Geometry check sheet. Reference: the model listing, model coordinates, mm. A direction names the side the tool comes from. Give positions to 0.01 mm unless a question says otherwise; leave off trailing zeros. Order: outer loops, then holes, each group sorted by start corner. A loop starts at its lowest first (then second) coordinate and runs counter-clockwise, first axis right, second up. Notation, with made-up numbers: (85, 47) - (124, 47) arc R36 ccw to (124, 85) - close; hole circle Ø6 at (31.25, -20.5). An arc over 180 degrees is marked (long way). Put each result on its own line as item: value. Start each with the question number.
Autodesk Inventor part; units mm, degrees
ref_plane "YZ Plane" through (0, 0, 0) normal (1, 0, 0) x (0, 1, 0)
ref_plane "XZ Plane" through (0, 0, 0) normal (0, 1, 0) x (-1, 0, 0)
ref_plane "XY Plane" through (0, 0, 0) normal (0, 0, 1) x (1, 0, 0)
sketch "Sketch1" plane through (0, 0, 0) normal (0, 0, 1) x (1, 0, 0)
  circle A0 centre (0, 0) radius 4
  circle A1 centre (0, 0) radius 50
  circle A2 centre (0, 0) radius 38
  dimension "d0" = 8
  dimension "d1" = 100
  dimension "d2" = 12
extrude "Extrusion1" add sketch "Sketch1" along normal blind 10 contours A1
sketch "Sketch2" plane through (0, 0, 10) normal (0, 0, 1) x (1, 0, 0)
  circle A0 centre (0, 0) radius 50
  circle A1 centre (0, 0) radius 4
  dimension "d5" = 8
  dimension "d6" = 100
sketch "Sketch3" plane through (0, 0, 10) normal (0, 0, 1) x (1, 0, 0)
  point P0 (0, 0)
extrude "Extrusion2" add sketch "Sketch2" along normal blind 6
sketch "Sketch4" plane through (0, 0, 16) normal (0, 0, 1) x (1, 0, 0)
  circle A0 centre (0, 0) radius 38
  circle A1 centre (0, 0) radius 50
  dimension "d9" = 76
  dimension "d10" = 100
extrude "Extrusion3" add sketch "Sketch4" along normal blind 10
sketch "Sketch5" plane through (0, 0, 16) normal (0, 0, 1) x (1, 0, 0)
  circle A0 centre (0, 0) radius 4
  circle A1 centre (0, 0) radius 6
  dimension "d13" = 8
  dimension "d14" = 12
extrude "Extrusion4" add sketch "Sketch5" along normal blind 20
properties part number "100mm wheel"
Item 1: Set-up check for faces 5 (the face through (-6, 0, 26)), 6 (the face through (17.535, 33.713, 4.93)), 7 (the face through (11, 37, 0)): record each of +Z, -Z, +X, -X, +Y, -Y from which the full face is reachable in a straight line by a thin tool's end or side.
Item 2: Cross-section at B-B (z = 22.5). Enter the section's corners in (x, y), and give its area (3 significant figures).
Item 3: Thickness scan on line 1 along Y through (x, z) = (0, 19.75); line 2 along Y through (x, z) = (0, 7.5); line 3 along Y through (x, z) = (0, 28). Record the ranges inside material, lowest first.
Item 4: Cross-section at D-D (y = 26.5). Enter the section's corners in (x, z), and give its area (3 significant figures).
Item 5: Release check for a two-part mould opening along Y. For faces 1 (the face through (17.535, 33.713, 20.93)), 2 (the face through (11, 37, 26)), 3 (the face through (47.69, -15.02, 12.82)), 4 (the face through (-1, -8, 10)) record: +Y half, -Y half, draft (parallel to the pull), parting line (faces both ways), or undercut.
Item 6: Cross-section at C-C (z = 7.5). Enter the section's corners in (x, y), and give its area (3 significant figures).
Item 7: Cross-section at A-A (x = 0). Enter the section's corners in (y, z), and give its area (3 significant figures).
Item 8: Gauge pin test, flat ends, axial feed: pin 1 Ø2 at (y, z) = (-23, 14) entering from +X; pin 2 Ø10 at (x, y) = (-27, -2.5) entering from -Z; pin 3 Ø6 at (x, z) = (6.5, 7.5) entering from +Y; pin 4 Ø7 at (x, y) = (0, 0) entering from +Z. Record the tip position at first contact, or that the pin passes through.
Recorded:
1. face 5: +Z
1. face 6: -Z
1. face 7: -Z, +X, -X, +Y, -Y
2. outline: circle Ø100 at (0, 0); circle Ø12 at (0, 0); hole circle Ø76 at (0, 0); hole circle Ø8 at (0, 0)
2. area: 3,380 mm^2
3. line 1: y = -50 to -38, -6 to -4, 4 to 6, 38 to 50
3. line 2: y = -50 to -38, 38 to 50
3. line 3: y = -6 to -4, 4 to 6
4. outline: (-42.4, 0) - (-27.24, 0) - (-27.24, 10) - (27.24, 10) - (27.24, 0) - (42.4, 0) - (42.4, 26) - (27.24, 26) - (27.24, 16) - (-27.24, 16) - (-27.24, 26) - (-42.4, 26) - close
4. area: 1,120 mm^2
5. face 1: undercut
5. face 2: draft
5. face 3: parting line
5. face 4: undercut
6. outline: circle Ø100 at (0, 0); hole circle Ø76 at (0, 0)
6. area: 3,320 mm^2
7. outline: (-50, 0) - (-38, 0) - (-38, 10) - (-4, 10) - (-4, 36) - (-6, 36) - (-6, 16) - (-38, 16) - (-38, 26) - (-50, 26) - close; (4, 10) - (38, 10) - (38, 0) - (50, 0) - (50, 26) - (38, 26) - (38, 16) - (6, 16) - (6, 36) - (4, 36) - close
7. area: 1,110 mm^2
8. pin 1: stops at x = 44.9
8. pin 2: stops at z = 10
8. pin 3: stops at y = 49.88
8. pin 4: passes through
